from build123d import *

# Parameters (mm, degrees)
SKETCH1_W           = 33
SKETCH1_H           = 13
BOSS_EXTRUDE1_DEPTH = 2
BOSS_EXTRUDE2_DEPTH = 1
FILLET1_R           = 0.5
SKETCH3_R           = 0.631168426
CUT_EXTRUDE1_DEPTH  = 0.1
FILLET2_R           = 0.04
SKETCH4_R           = 0.625
BOSS_EXTRUDE3_DEPTH = 0.6
BOSS_EXTRUDE3_TAPER = 27


with BuildPart() as part:
    # Sketch1 → Boss-Extrude1 (new body)
    with BuildSketch(Plane(origin=(0, 0, 0), x_dir=(1, 0, 0), z_dir=(0, 1, 0))):
        Rectangle(SKETCH1_W, SKETCH1_H)
    extrude(amount=BOSS_EXTRUDE1_DEPTH)

    # Sketch2 → Boss-Extrude2 (add)
    with BuildSketch(Plane(origin=(0, 2, 0), x_dir=(1, 0, 0), z_dir=(0, 1, 0))):
        Polygon((-11.063698409, -0.221797323), (-5.897125464, -4.944775622), (-1.174147166, 0.221797323), (-6.340720111, 4.944775622), align=None)
    extrude(amount=BOSS_EXTRUDE2_DEPTH)

    # Fillet1
    fillet1_edges = [part.edges().sort_by_distance(p)[0] for p in [
        (-8.70220926, 3, -2.361489149),
        (-8.480411937, 3, 2.583286472),
        (-3.535636315, 3, 2.361489149),
        (-3.757433638, 3, -2.583286472),
    ]]
    fillet(fillet1_edges, radius=FILLET1_R)

    # Sketch3 → Cut-Extrude1 (cut)
    with BuildSketch(Plane(origin=(0, 3, 0), x_dir=(1, 0, 0), z_dir=(0, 1, 0))):
        with Locations(Location((-2.868853152, 0.151489879, 0), (0, 0, 270))):
            Circle(SKETCH3_R)
    extrude(amount=-CUT_EXTRUDE1_DEPTH, mode=Mode.SUBTRACT)

    # Fillet2
    fillet2_edges = [part.edges().sort_by_distance(p)[0] for p in [
        (-2.868853152, 3, -0.782658305),
    ]]
    fillet(fillet2_edges, radius=FILLET2_R)

    # Sketch4 → Boss-Extrude3 (add)
    with BuildSketch(Plane(origin=(0, 2, 0), x_dir=(1, 0, 0), z_dir=(0, 1, 0))):
        with Locations((-13.5, 5.5)):
            Circle(SKETCH4_R)
        with Locations((-11.25, 5.5)):
            Circle(SKETCH4_R)
        with Locations((-9, 5.5)):
            Circle(SKETCH4_R)
        with Locations((-6.75, 5.5)):
            Circle(SKETCH4_R)
        with Locations((-4.5, 5.5)):
            Circle(SKETCH4_R)
        with Locations((-2.25, 5.5)):
            Circle(SKETCH4_R)
        with Locations((0, 5.5)):
            Circle(SKETCH4_R)
        with Locations((2.25, 5.5)):
            Circle(SKETCH4_R)
        with Locations((4.5, 5.5)):
            Circle(SKETCH4_R)
        with Locations((6.75, 5.5)):
            Circle(SKETCH4_R)
        with Locations((9, 5.5)):
            Circle(SKETCH4_R)
        with Locations((11.25, 5.5)):
            Circle(SKETCH4_R)
        with Locations((13.5, 5.5)):
            Circle(SKETCH4_R)
        with Locations((-13.5, -5.5)):
            Circle(SKETCH4_R)
        with Locations((-11.25, -5.5)):
            Circle(SKETCH4_R)
        with Locations((-9, -5.5)):
            Circle(SKETCH4_R)
        with Locations((-6.75, -5.5)):
            Circle(SKETCH4_R)
        with Locations((-4.5, -5.5)):
            Circle(SKETCH4_R)
        with Locations((-2.25, -5.5)):
            Circle(SKETCH4_R)
        with Locations((0, -5.5)):
            Circle(SKETCH4_R)
        with Locations((2.25, -5.5)):
            Circle(SKETCH4_R)
        with Locations((4.5, -5.5)):
            Circle(SKETCH4_R)
        with Locations((6.75, -5.5)):
            Circle(SKETCH4_R)
        with Locations((9, -5.5)):
            Circle(SKETCH4_R)
        with Locations((11.25, -5.5)):
            Circle(SKETCH4_R)
        with Locations((13.5, -5.5)):
            Circle(SKETCH4_R)
    extrude(amount=BOSS_EXTRUDE3_DEPTH, taper=BOSS_EXTRUDE3_TAPER)


solid = part.part
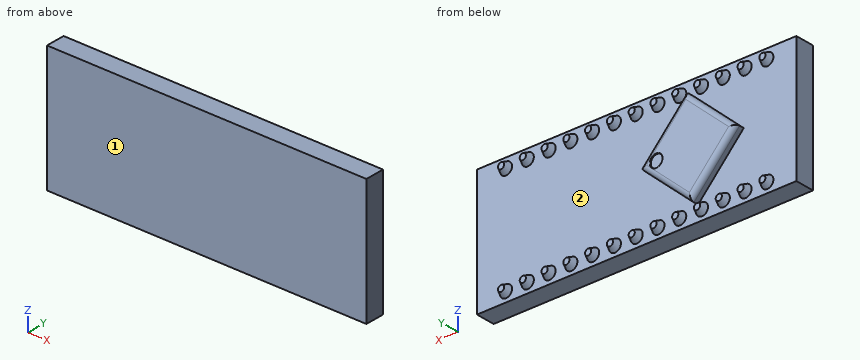
Design review of the part built by this model. Coordinates are the model's own, in mm. Face numbers are marked on the shaded views. Coordinates: 2 decimals unless noted, no trailing zeros. Loops run counter-clockwise (first coordinate to the right, second up) from the corner with the lowest first, then second, coordinate; pieces in that order, holes last. Notation, with made-up numbers: (78.25, 65) - (93.25, 65) arc R35 cw to (93.25, 103) - close; hole circle Ø7 at (24.25, 76.5). An arc over 180 degrees is marked (long way). Use CSV: the item, a comma, the result in double quotes. Start each with the question number.
1. Add section B-B on x = 5.5. Give the boundary of the cut face in (y, z), plus the area to 3 significant figures.
2. To check wall thickness, follow probe 1 along Z at (x, y) = (-2.5, 2.5); probe 2 along Y at (x, z) = (3.5, 4.75); probe 3 along Z at (x, y) = (-9, 2.35). State the ranges of each line that lie inside material, in increasing order.
3. Add section A-A on x = -13.5. Give the boundary of the cut face in (y, z) (3 decimals).
4. Clearance check with flat-ended pins moving along their axes: pin 1 (6 mm diameter, centred on x = 8.5, z = -1, fed in from +Y); pin 2 (0.5 mm diameter, centred on x = 13.5, z = -5.5, fed in from +Y). State where each tip first meets the part, or that it passes through.
5. Mouldability with a two-part tool opening along Z and no side actions: class the marked faces 1 and 2 as released by +Z, released by -Z, zero draft, split by the parting line, or undercut.
Resolved:
1,outline,"(0, -6.5) - (2, -6.5) - (2, 6.5) - (0, 6.5) - close"
1,area,"26.0 mm2"
2,probe 1,"-5.77 to -5.23, -1.43 to 1.23, 5.23 to 5.77"
2,probe 2,"0 to 2"
2,probe 3,"-5.95 to -5.05, -2.04 to 2.11, 5.05 to 5.95"
3,outline,"(0, -6.5) - (2, -6.5) - (2, -6.125) - (2.6, -5.819) - (2.6, -5.181) - (2, -4.875) - (2, 4.875) - (2.6, 5.181) - (2.6, 5.819) - (2, 6.125) - (2, 6.5) - (0, 6.5) - close"
4,pin 1,"y = 2"
4,pin 2,"y = 2.6"
5,face 1,"zero draft"
5,face 2,"undercut"
